For this review, take the finished solid that the model builds, in its own axes (mm). Give positions to 0.01 mm unless a question says otherwise; leave off trailing zeros. Write each loop counter-clockwise with the first axis right and the second up, starting at its lowest first coordinate (ties: lowest second). Pieces come first, ordered by that corner, then holes. Notation, with made-up numbers: M -38,27.25 L -23,27.25 A26 ccw -23,54.25 Z; hole C -35,37 d3. An arc over 180 degrees is marked long. Answer as a JSON object with one key per item and string values. Group by question number.
```python
from build123d import *

# Parameters (mm, degrees)
BASE_W_MOTOR_MOUNTS_R  = 70
BOSS_EXTRUDE1_DEPTH    = 3.175
STANDOFFS_TOP_BOTTOM_R = 1.65
CUT_EXTRUDE2_DEPTH     = 3.175


with BuildPart() as part:
    # Base w/ Motor Mounts → Boss-Extrude1 (new body)
    with BuildSketch(Plane(origin=(0, 0, 0), x_dir=(1, 0, 0), z_dir=(0, 1, 0))):
        Circle(BASE_W_MOTOR_MOUNTS_R)
    extrude(amount=BOSS_EXTRUDE1_DEPTH)

    # Standoffs (top / bottom) → Cut-Extrude2 (cut)
    with BuildSketch(Plane(origin=(0, 0, 0), x_dir=(1, 0, 0), z_dir=(0, 1, 0))):
        with Locations((60.976049146, 25.257106536)):
            Circle(STANDOFFS_TOP_BOTTOM_R)
        with Locations((60.976049146, -25.257106536)):
            Circle(STANDOFFS_TOP_BOTTOM_R)
        with Locations((-60.976049146, -25.257106536)):
            Circle(STANDOFFS_TOP_BOTTOM_R)
        with Locations((-60.976049146, 25.257106536)):
            Circle(STANDOFFS_TOP_BOTTOM_R)
        with Locations((10.5, -60.953059289)):
            Circle(STANDOFFS_TOP_BOTTOM_R)
        with Locations((-10.5, -60.953059289)):
            Circle(STANDOFFS_TOP_BOTTOM_R)
    extrude(amount=CUT_EXTRUDE2_DEPTH, mode=Mode.SUBTRACT)


solid = part.part
```
Item 1: Consider section D-D (x = 19.5). Give the boundary of the cut face in (y, z) (3 decimals), plus the area to 3 significant figures.
Item 2: Consider section A-A (x = -10.5). Give the boundary of the cut face in (y, z) (3 decimals).
Item 3: Draft analysis for pull direction Z (two halves, no side actions). For faces 1 (the flat face through (-1, 3.175, -1)), 2 (the cylindrical face through (-10.858, 1.565, 62.564)), 3 (the cylindrical face through (-55.55, 1.565, 42.594)), state which applies: released by +Z, released by -Z, zero draft, split by the parting line, or undercut.
Item 4: To check wall thickness, follow probe 1 along X at (y, z) = (2.95, 60.5); probe 2 along Z at (x, y) = (61, 1.2); probe 3 along Z at (x, y) = (2, 0.25). State the ranges of each line that lie inside material, in increasing order.
Item 5: Consider section C-C (x = -56). Give the boundary of the cut face in (y, z) (3 decimals).
Item 6: Consider section B-B (y = 1.7). Give the boundary of the cut face in (x, z), plus the area to 3 significant figures.
Item 7: Insertion check: P1, Ø2, axis at x = 60.98, z = 25.26, coming from the -Y side. The pin has a flat end and moves straight along its axis. Give the tip position at first contact, or say it passes through.
Result set:
{
 "1": {"outline": "M 0,-67.229 L 3.175,-67.229 L 3.175,67.229 L 0,67.229 Z", "area": "427 mm^2"},
 "2": {"outline": "M 0,-69.208 L 3.175,-69.208 L 3.175,59.303 L 0,59.303 Z; M 0,62.603 L 3.175,62.603 L 3.175,69.208 L 0,69.208 Z"},
 "3": {"face 1": "zero draft", "face 2": "undercut", "face 3": "split by the parting line"},
 "4": {"probe 1": "x = -35.21 to -12.09, -8.91 to 8.91, 12.09 to 35.21", "probe 2": "z = -34.34 to -26.91, -23.61 to 23.61, 26.91 to 34.34", "probe 3": "z = -69.97 to 69.97"},
 "5": {"outline": "M 0,-42 L 3.175,-42 L 3.175,42 L 0,42 Z"},
 "6": {"outline": "C 0,0 d140; hole C -60.98,-25.26 d3.3; hole C -60.98,25.26 d3.3; hole C -10.5,60.95 d3.3; hole C 10.5,60.95 d3.3; hole C 60.98,-25.26 d3.3; hole C 60.98,25.26 d3.3", "area": "15,300 mm^2"},
 "7": {"P1": "passes through"}
}
